The model under review builds one solid part; all positions refer to its coordinate system, in mm. Face numbers are marked on the shaded views. A direction names the side the tool comes from. Give positions to 0.01 mm unless a question says otherwise; leave off trailing zeros. Order: outer loops, then holes, each group sorted by start corner. A loop starts at its lowest first (then second) coordinate and runs counter-clockwise, first axis right, second up. Notation, with made-up numbers: (76.5, 8) -> (93.5, 8) arc R26 ccw to (93.5, 47) -> close; hole circle Ø4 at (11, -29.5). An arc over 180 degrees is marked (long way). Use one line per item in the form item = value.
```python
from build123d import *

# Parameters (mm, degrees)
CYLINDER008_R     = 5.5
CYLINDER008_DEPTH = 2
FILLET005_R       = 1
CYLINDER009_R     = 5.5
CYLINDER009_DEPTH = 2
FILLET006_R       = 1
CYLINDER006_R     = 5.5
CYLINDER006_DEPTH = 2
FILLET003_R       = 1
CYLINDER007_R     = 5.5
CYLINDER007_DEPTH = 2
FILLET004_R       = 1
BOX001_W          = 35.5
BOX001_H          = 35.5
BOX001_DEPTH      = 7
FILLET_R          = 1.5
PRISM_DEPTH       = 12
CYLINDER_R        = 10
CYLINDER_DEPTH    = 12
BOX_W             = 40
BOX_H             = 40
BOX_DEPTH         = 10
FILLET001_R       = 2


with BuildPart() as fillet005:
    # Cylinder008 → Cylinder008 (new body)
    with BuildSketch(Plane.XY):
        Circle(CYLINDER008_R)
    extrude(amount=CYLINDER008_DEPTH)

    # Fillet005
    fillet005_edges = [fillet005.edges().sort_by_distance(p)[0] for p in [
        (-5.5, 0, 2),
    ]]
    fillet(fillet005_edges, radius=FILLET005_R)


with BuildPart() as fillet005_1:
    # Fillet005 placement: moved
    add(fillet005.part.moved(Location((10, 30, 7))))


with BuildPart() as fillet006:
    # Cylinder009 → Cylinder009 (new body)
    with BuildSketch(Plane.XY):
        Circle(CYLINDER009_R)
    extrude(amount=CYLINDER009_DEPTH)

    # Fillet006
    fillet006_edges = [fillet006.edges().sort_by_distance(p)[0] for p in [
        (-5.5, 0, 2),
    ]]
    fillet(fillet006_edges, radius=FILLET006_R)


with BuildPart() as fillet006_1:
    # Fillet006 placement: moved
    add(fillet006.part.moved(Location((30, 30, 7))))


with BuildPart() as fillet003:
    # Cylinder006 → Cylinder006 (new body)
    with BuildSketch(Plane.XY):
        Circle(CYLINDER006_R)
    extrude(amount=CYLINDER006_DEPTH)

    # Fillet003
    fillet003_edges = [fillet003.edges().sort_by_distance(p)[0] for p in [
        (-5.5, 0, 2),
    ]]
    fillet(fillet003_edges, radius=FILLET003_R)


with BuildPart() as fillet003_1:
    # Fillet003 placement: moved
    add(fillet003.part.moved(Location((10, 10, 7))))


with BuildPart() as fillet004:
    # Cylinder007 → Cylinder007 (new body)
    with BuildSketch(Plane.XY):
        Circle(CYLINDER007_R)
    extrude(amount=CYLINDER007_DEPTH)

    # Fillet004
    fillet004_edges = [fillet004.edges().sort_by_distance(p)[0] for p in [
        (-5.5, 0, 2),
    ]]
    fillet(fillet004_edges, radius=FILLET004_R)


with BuildPart() as fillet004_1:
    # Fillet004 placement: moved
    add(fillet004.part.moved(Location((30, 10, 7))))


with BuildPart() as fillet_body:
    # Box001 → Box001 (new body)
    with BuildSketch(Plane(origin=(2.25, 2.25, 0), x_dir=(1, 0, 0), z_dir=(0, 0, 1))):
        with Locations((17.75, 17.75)):
            Rectangle(BOX001_W, BOX001_H)
    extrude(amount=BOX001_DEPTH)

    # Fillet
    fillet_edges = [fillet_body.edges().sort_by_distance(p)[0] for p in [
        (2.25, 2.25, 3.5),
        (2.25, 37.75, 3.5),
        (37.75, 2.25, 3.5),
        (37.75, 37.75, 3.5),
    ]]
    fillet(fillet_edges, radius=FILLET_R)


with BuildPart() as prism:
    # Prism → Prism (new body)
    with BuildSketch(Plane(origin=(20, 20, 0), x_dir=(1, 0, 0), z_dir=(0, 0, 1))):
        Polygon((7.505, 0), (3.7525, 6.499521), (-3.7525, 6.499521), (-7.505, 0), (-3.7525, -6.499521), (3.7525, -6.499521), align=None)
    extrude(amount=PRISM_DEPTH)


with BuildPart() as cylinder:
    # Cylinder → Cylinder (new body)
    with BuildSketch(Plane(origin=(20, 20, 0), x_dir=(1, 0, 0), z_dir=(0, 0, 1))):
        Circle(CYLINDER_R)
    extrude(amount=CYLINDER_DEPTH)


with BuildPart() as cut010:
    # Box → Box (new body)
    with BuildSketch(Plane.XY):
        with Locations((20, 20)):
            Rectangle(BOX_W, BOX_H)
    extrude(amount=BOX_DEPTH)

    # Fusion: union Cylinder
    add(cylinder.part)

    # Cut: cut Prism
    add(prism.part, mode=Mode.SUBTRACT)

    # Fillet001
    fillet001_edges = [cut010.edges().sort_by_distance(p)[0] for p in [
        (0, 0, 5),
        (0, 20, 10),
        (0, 40, 5),
        (40, 0, 5),
        (20, 0, 10),
        (20, 40, 10),
        (40, 20, 10),
        (40, 40, 5),
    ]]
    fillet(fillet001_edges, radius=FILLET001_R)

    # Cut001: cut Fillet body
    add(fillet_body.part, mode=Mode.SUBTRACT)

    # Cut007: cut Fillet004
    add(fillet004_1.part, mode=Mode.SUBTRACT)

    # Cut008: cut Fillet003
    add(fillet003_1.part, mode=Mode.SUBTRACT)

    # Cut009: cut Fillet006
    add(fillet006_1.part, mode=Mode.SUBTRACT)

    # Cut010: cut Fillet005
    add(fillet005_1.part, mode=Mode.SUBTRACT)


solid = cut010.part
```
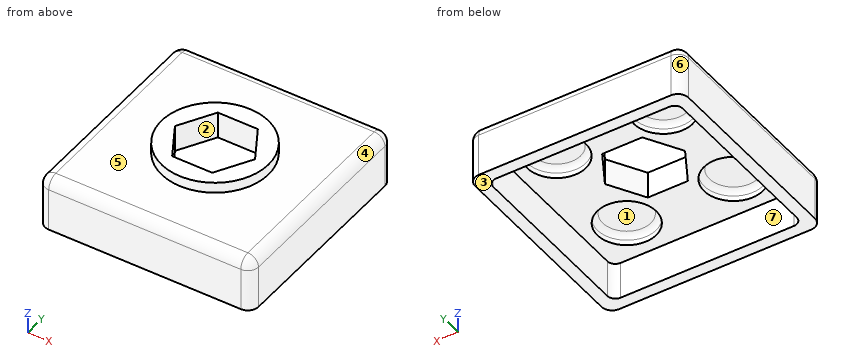
1. Add section B-B on x = 20. Give the boundary of the cut face in (y, z).
Values:
outline = (0, 0) -> (2.25, 0) -> (2.25, 7) -> (13.5, 7) -> (13.5, 12) -> (10, 12) -> (10, 10) -> (2, 10) arc R2 ccw to (0, 8) -> close; (26.5, 7) -> (37.75, 7) -> (37.75, 0) -> (40, 0) -> (40, 8) arc R2 ccw to (38, 10) -> (30, 10) -> (30, 12) -> (26.5, 12) -> close
2. The part is to be moulded in two halves that separate along X. For the marked faces 4, 5, 6 and 7, say which applies: +X half, -X half, draft (parallel to the pull), parting line (faces both ways), or undercut.
Values:
face_4 = +X half
face_5 = draft
face_6 = -X half
face_7 = undercut
3. Add section C-C on z = 7.5. Give the boundary of the cut face in (x, y) (1 decimal).
Values:
outline = (0, 2) arc R2 ccw to (2, 0) -> (38, 0) arc R2 ccw to (40, 2) -> (40, 38) arc R2 ccw to (38, 40) -> (2, 40) arc R2 ccw to (0, 38) -> close; hole circle Ø11 at (10, 10); hole circle Ø11 at (10, 30); hole (12.5, 20) -> (16.2, 13.5) -> (23.8, 13.5) -> (27.5, 20) -> (23.8, 26.5) -> (16.2, 26.5) -> close; hole circle Ø11 at (30, 10); hole circle Ø11 at (30, 30)
4. Add section A-A on z = 3.5. Give the boundary of the cut face in (x, y).
Values:
outline = (0, 2) arc R2 ccw to (2, 0) -> (38, 0) arc R2 ccw to (40, 2) -> (40, 38) arc R2 ccw to (38, 40) -> (2, 40) arc R2 ccw to (0, 38) -> close; hole (2.25, 3.75) arc R1.5 ccw to (3.75, 2.25) -> (36.25, 2.25) arc R1.5 ccw to (37.75, 3.75) -> (37.75, 36.25) arc R1.5 ccw to (36.25, 37.75) -> (3.75, 37.75) arc R1.5 ccw to (2.25, 36.25) -> close
5. Tool access review of the marked faces 1, 2 and 3: name each direction out of +Z, -Z, +X, -X, +Y, -Y from which nothing blocks a thin tool from reaching the whole face with its end or side.
Values:
face_1 = -Z
face_2 = +Z, -Z
face_3 = -Z, +X, -X, +Y, -Y
6. For pin 1 Ø1 at (x, y) = (10, 10.5) entering from -Z; pin 2 Ø1.5 at (x, z) = (20.5, 10) entering from +Y; pin 3 Ø1.5 at (x, z) = (21, 9.5) entering from -Y, all flat-tipped, find the tip position at first contact; note any pin that passes through.
Values:
pin_1 = 9
pin_2 = 39.56
pin_3 = 0.15
7. For L1, parallel to Y at x = 35.5, z = 1.75; L2, parallel to Y at x = 30, z = 7.3; L3, parallel to X at y = 29, z = 7.75, list the stretches that pass through material, from the lowest coordinate up.
Values:
L1 = 0 to 2.25, 37.75 to 40
L2 = 0 to 4.5, 15.5 to 24.5, 35.5 to 40
L3 = 0 to 4.59, 15.41 to 24.59, 35.41 to 40
